```python
from build123d import *

# Parameters (mm, degrees)
SKETCH1_R           = 38.1
BOSS_EXTRUDE1_DEPTH = 6.35
SKETCH4_W           = 25.4
SKETCH4_H           = 25.4
BOSS_EXTRUDE2_DEPTH = 228.6
SKETCH5_W           = 22.225
SKETCH5_H           = 22.225
CUT_EXTRUDE1_DEPTH  = 228.6
SKETCH8_W           = 12.7
SKETCH8_H           = 25.4
CUT_EXTRUDE2_DEPTH  = 25.4
SKETCH7_W           = 12.7
SKETCH7_H           = 12.7
BOSS_EXTRUDE4_DEPTH = 203.2
SKETCH9_W           = 46.99
SKETCH9_H           = 55.88
BOSS_EXTRUDE5_DEPTH = 6.35


with BuildPart() as part:
    # Sketch1 → Boss-Extrude1 (new body)
    with BuildSketch(Plane(origin=(0, 0, 0), x_dir=(1, 0, 0), z_dir=(0, 1, 0))):
        Circle(SKETCH1_R)
    extrude(amount=BOSS_EXTRUDE1_DEPTH)

    # Sketch4 → Boss-Extrude2 (add)
    with BuildSketch(Plane(origin=(0, 6.35, 0), x_dir=(1, 0, 0), z_dir=(0, 1, 0))):
        Rectangle(SKETCH4_W, SKETCH4_H)
    extrude(amount=BOSS_EXTRUDE2_DEPTH)

    # Sketch5 → Cut-Extrude1 (cut)
    with BuildSketch(Plane(origin=(0, 234.95, 0), x_dir=(1, 0, 0), z_dir=(0, 1, 0))):
        Rectangle(SKETCH5_W, SKETCH5_H)
    extrude(amount=-CUT_EXTRUDE1_DEPTH, mode=Mode.SUBTRACT)

    # Sketch8 → Cut-Extrude2 (cut)
    with BuildSketch(Plane.XY.offset(12.7)):
        with Locations((6.35, 19.05)):
            Rectangle(SKETCH8_W, SKETCH8_H)
    extrude(amount=-CUT_EXTRUDE2_DEPTH, mode=Mode.SUBTRACT)

    # Sketch7 → Boss-Extrude4 (add)
    with BuildSketch(Plane(origin=(0, 6.35, 0), x_dir=(1, 0, 0), z_dir=(0, 1, 0))):
        Rectangle(SKETCH7_W, SKETCH7_H)
    extrude(amount=BOSS_EXTRUDE4_DEPTH)

    # Sketch9 → Boss-Extrude5 (add)
    with BuildSketch(Plane.XZ):
        with Locations((23.495, 27.94)):
            Rectangle(SKETCH9_W, SKETCH9_H)
    extrude(amount=-BOSS_EXTRUDE5_DEPTH)


solid = part.part
```
Geometry: final body of the model. Coordinates: model frame, mm. A direction names the side the tool comes from. Round coordinates to 2 decimals unless told otherwise and drop trailing zeros. Write each loop counter-clockwise with the first axis right and the second up, starting at its lowest first coordinate (ties: lowest second). Pieces come first, ordered by that corner, then holes.
Item 1: Pin query (flat end, axial travel): P1, Ø24.5, axis at y = 111, z = 3, coming from the -X side; P2, Ø7, axis at y = 2.5, z = 49.5, coming from the -X side; P3, Ø0.8, axis at y = 23, z = 12, coming from the +X side. Return the tip coordinate at first contact, or that it passes through.
Item 2: Section query A-A (y = 113.5). Return loops of the section in (x, z), plus the area to 4 significant figures.
Item 3: Set-up query: faces 1 (the face through (0, 119, 12.7)), 2 (the face through (11.112, 135, 0)), 3 (the face through (-12.7, 119, 0)), 4 (the face through (42, 3, 0)), 5 (the face through (0, 119, -12.7)). Return all of +Z, -Z, +X, -X, +Y, -Y with unobstructed straight access to the full face (end or side cutting, diameter ignored); none if empty.
Item 4: Section query B-B (y = 24.5). Return loops of the section in (x, z), plus the area to 3 significant figures.
Item 5: Section query C-C (x = -15). Return loops of the section in (y, z), plus the area to 3 significant figures.
Item 6: Section query D-D (z = 20). Return loops of the section in (x, y).
Item 7: Material intervals for L1, parallel to Z at x = 4, y = 56; L2, parallel to X at y = 81, z = -7.5, sorted ascending.
Item 8: Mould query, pull axis Y, two halves, no side actions, for faces 6 (the face through (46.99, 3, 28)), 7 (the face through (11.5, 31.75, 1)), 8 (the face through (0, 209.55, 0)). Classes: +Y half, -Y half, draft (parallel to the pull), parting line (faces both ways), or undercut.
Completed:
1. P1: stops at x = -12.7
1. P2: stops at x = 0
1. P3: stops at x = 0
2. outline: (-12.7, -12.7) - (12.7, -12.7) - (12.7, 12.7) - (-12.7, 12.7) - close; (-6.35, -6.35) - (6.35, -6.35) - (6.35, 6.35) - (-6.35, 6.35) - close; hole (-11.11, -11.11) - (11.11, -11.11) - (11.11, 11.11) - (-11.11, 11.11) - close
2. area: 312.5 mm2
3. face 1: +Z, +X, -X, +Y
3. face 2: +Y
3. face 3: +Z, -Z, -X, +Y
3. face 4: -Z, +X, +Y, -Y
3. face 5: -Z, +X, -X, +Y
4. outline: (-12.7, -12.7) - (0, -12.7) - (0, -11.11) - (-11.11, -11.11) - (-11.11, 11.11) - (0, 11.11) - (0, 12.7) - (-12.7, 12.7) - close; (-6.35, -6.35) - (6.35, -6.35) - (6.35, 6.35) - (-6.35, 6.35) - close
4. area: 237 mm2
5. outline: (0, -35.02) - (6.35, -35.02) - (6.35, 35.02) - (0, 35.02) - close
5. area: 445 mm2
6. outline: (-32.43, 0) - (46.99, 0) - (46.99, 6.35) - (-32.43, 6.35) - close
7. L1: z = -12.7 to -11.11, -6.35 to 6.35, 11.11 to 12.7
7. L2: x = -12.7 to -11.11, 11.11 to 12.7
8. face 6: draft
8. face 7: undercut
8. face 8: +Y half
